Work out the finished part from the listing and answer in its coordinate system (mm). Face numbers are marked on the shaded views. A direction names the side the tool comes from. Coordinates: 2 decimals unless noted, no trailing zeros. Order: outer loops, then holes, each group sorted by start corner. A loop starts at its lowest first (then second) coordinate and runs counter-clockwise, first axis right, second up. Notation, with made-up numbers: M 40.25,43 L 63.25,43 A8 ccw 63.25,53 Z; hole C 53,-39.5 d7. An arc over 180 degrees is marked long. Use a Markdown table: item, result.
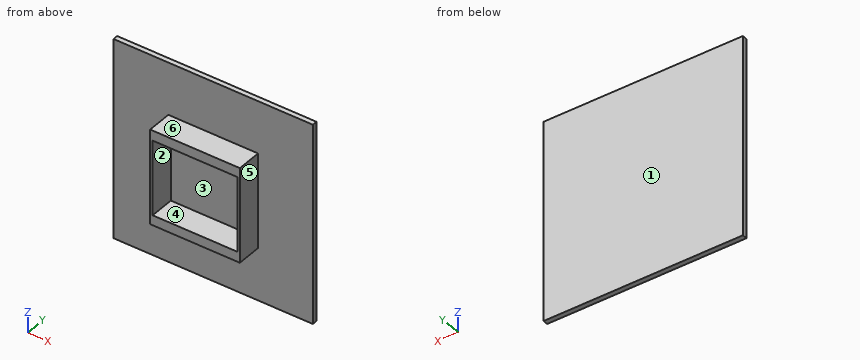
from build123d import *

# Parameters (mm, degrees)
BASE_DEPTH          = 2.5
BASE_DEPTH_BACK     = 2.5
SKETCH1_W           = 200
SKETCH1_H           = 200
SKETCH2_W           = 90
SKETCH2_H           = 95
SKETCH2_W_2         = 85
SKETCH2_H_2         = 75
BATTERYHOLDER_DEPTH = 25


with BuildPart() as part:
    # Sketch1 → Base (new, two sides: drawn at the far end of the back side and taken through both)
    with BuildSketch(Plane(origin=(0, 0, 0), x_dir=(1, 0, 0), z_dir=(0, 1, 0)).offset(-BASE_DEPTH_BACK)):
        Rectangle(SKETCH1_W, SKETCH1_H)
    extrude(amount=BASE_DEPTH + BASE_DEPTH_BACK)

    # Sketch2 → BatteryHolder (add)
    with BuildSketch(Plane(origin=(0, -2.5, 0), x_dir=(-1, 0, 0), z_dir=(0, -1, 0))):
        Rectangle(SKETCH2_W, SKETCH2_H)
        Rectangle(SKETCH2_W_2, SKETCH2_H_2, mode=Mode.SUBTRACT)
    extrude(amount=BATTERYHOLDER_DEPTH)


solid = part.part
1. For a pull along Z with two mould halves and no side action, classify the marked faces 3, 4, 5 and 6 as +Z half, -Z half, draft (parallel to the pull), parting line (faces both ways), or undercut.
Answers below:
| item | result |
|---|---|
| face 3 | undercut |
| face 4 | undercut |
| face 5 | draft |
| face 6 | +Z half |
2. Section A-A on y = -20.5 is taken. Determine the outline of the cut face in (x, z), then the cut area to 4 significant figures.
Answers below:
| item | result |
|---|---|
| outline | M -45,-47.5 L 45,-47.5 L 45,47.5 L -45,47.5 Z; hole M -42.5,-37.5 L 42.5,-37.5 L 42.5,37.5 L -42.5,37.5 Z |
| area | 2,175 mm² |
3. Section C-C on x = -32.5 is taken. Determine the outline of the cut face in (y, z).
Answers below:
| item | result |
|---|---|
| outline | M -27.5,-47.5 L -2.5,-47.5 L -2.5,-100 L 2.5,-100 L 2.5,100 L -2.5,100 L -2.5,47.5 L -27.5,47.5 L -27.5,37.5 L -2.5,37.5 L -2.5,-37.5 L -27.5,-37.5 Z |
4. Flat-ended cylindrical pins translate along their axes: P1, Ø7.5, axis at x = 22, y = -17.5, coming from the -Z side; P2, Ø5, axis at y = -12.5, z = -49.5, coming from the +X side; P3, Ø5, axis at x = -14.5, y = -16, coming from the +Z side. Find the tip coordinate at first contact, or state that the pin passes through.
Answers below:
| item | result |
|---|---|
| P1 | z = -47.5 |
| P2 | x = 45 |
| P3 | z = 47.5 |
5. Section B-B on z = -29 is taken. Determine the outline of the cut face in (x, y).
Answers below:
| item | result |
|---|---|
| outline | M -100,-2.5 L -45,-2.5 L -45,-27.5 L -42.5,-27.5 L -42.5,-2.5 L 42.5,-2.5 L 42.5,-27.5 L 45,-27.5 L 45,-2.5 L 100,-2.5 L 100,2.5 L -100,2.5 Z |
6. For the marked faces 1 and 2, determine the directions among +Z, -Z, +X, -X, +Y, -Y from which every point of the face is accessible in a straight line to the end or side of a thin tool.
Answers below:
| item | result |
|---|---|
| face 1 | +Z, -Z, +X, -X, +Y |
| face 2 | -Y |
7. Find the intervals of material crossed by probe 1 along X at (y, z) = (-17.5, 2.5); probe 2 along Z at (x, y) = (-39, -10.5); probe 3 along Y at (x, z) = (69.5, -89), in increasing order.
Answers below:
| item | result |
|---|---|
| probe 1 | -45 to -42.5, 42.5 to 45 |
| probe 2 | -47.5 to -37.5, 37.5 to 47.5 |
| probe 3 | -2.5 to 2.5 |
8. Section D-D on x = 66.5 is taken. Determine the outline of the cut face in (y, z).
Answers below:
| item | result |
|---|---|
| outline | M -2.5,-100 L 2.5,-100 L 2.5,100 L -2.5,100 Z |
